Work out the finished part from the listing and answer in its coordinate system (mm). Face numbers are marked on the shaded views. A direction names the side the tool comes from. Coordinates: 2 decimals unless noted, no trailing zeros. Order: outer loops, then holes, each group sorted by start corner. A loop starts at its lowest first (then second) coordinate and runs counter-clockwise, first axis right, second up. Notation, with made-up numbers: M 31,85 L 87,85 A31 ccw 87,114 Z; hole C 0.5,33.25 d4. An arc over 180 degrees is marked long. Write item = value, one per line. Start each with the question number.
Q1. Determine the mould class of the marked faces 3, 4 and 5 for opening direction X: released by +X, released by -X, zero draft, split by the parting line, or undercut.
Q2. Find section B-B on z = -11.5. Give the vertices of the cut face in (x, y), and give its area (3 significant figures).
Q3. Find section A-A on y = 11. Give the vertices of the cut face in (x, z), and give its area (3 significant figures).
Q4. A tool of negligible diameter and unlimited length cuts with its end or side. For the marked faces 1 and 2, from which of +Z, -Z, +X, -X, +Y, -Y can it reach the whole face along a straight path? Write none if from no direction.
Q5. Find section C-C on x = 5.25. Give the vertices of the cut face in (y, z), and give its area (3 significant figures).
Q6. Straight lines are drawn through the part: line 1 along X through (y, z) = (15, -10.75); line 2 along Z through (x, y) = (4.5, 17.25); line 3 along Y through (x, z) = (9.25, -7.5). For each, find the intervals that lie inside material, in ascending order.
Q7. This flat-tipped pin is pushed along its axis until it touches: P1, Ø1.5, axis at x = 4, y = 3, coming from the +Z side. Where does it stop, or does it pass through?
Q8. Find section D-D on x = 2.75. Give the vertices of the cut face in (y, z), and give its area (3 significant figures).
```python
from build123d import *

# Parameters (mm, degrees)
SKETCH1_W           = 12
SKETCH1_H           = 16
BOSS_EXTRUDE1_DEPTH = 18
SHELL1_T            = -2
SKETCH2_R           = 0.75
CUT_EXTRUDE1_DEPTH  = 10


with BuildPart() as part:
    # Sketch1 → Boss-Extrude1 (new body)
    with BuildSketch(Plane(origin=(0, 0, 0), x_dir=(1, 0, 0), z_dir=(0, 1, 0))):
        with Locations((6, 8)):
            Rectangle(SKETCH1_W, SKETCH1_H)
    extrude(amount=BOSS_EXTRUDE1_DEPTH)

    # Shell1
    shell1_openings = [part.faces().sort_by_distance(p)[0] for p in [
        (6, 18, -8),
    ]]
    offset(amount=SHELL1_T, openings=shell1_openings, kind=Kind.INTERSECTION)

    # Sketch2 → Cut-Extrude1 (cut)
    with BuildSketch(Plane.XZ):
        with Locations((4.770114722, -4.163836206)):
            Circle(SKETCH2_R)
        with Locations((4.770114722, -6.703836206)):
            Circle(SKETCH2_R)
        with Locations((4.770114721, -11.783836206)):
            Circle(SKETCH2_R)
    extrude(amount=-CUT_EXTRUDE1_DEPTH, mode=Mode.SUBTRACT)


solid = part.part
```
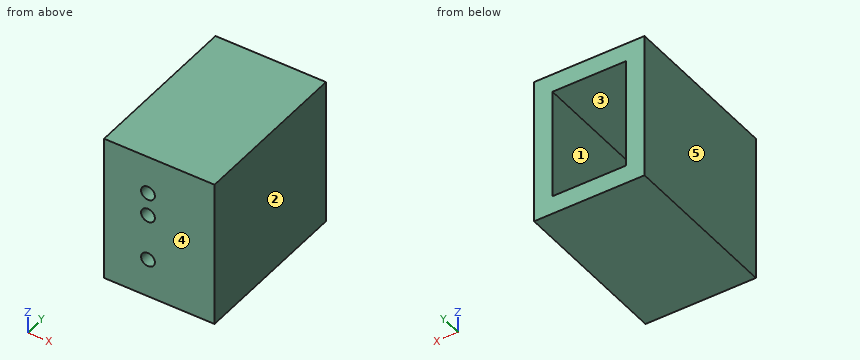
Findings below:
q1.face_3 = undercut
q1.face_4 = zero draft
q1.face_5 = released by -X
q2.outline = M 0,0 L 4.08,0 L 4.08,2 L 2,2 L 2,18 L 0,18 Z; M 5.46,0 L 12,0 L 12,18 L 10,18 L 10,2 L 5.46,2 Z
q2.area = 85.2 mm^2
q3.outline = M 0,-16 L 12,-16 L 12,0 L 0,0 Z; hole M 2,-14 L 10,-14 L 10,-2 L 2,-2 Z
q3.area = 96.0 mm^2
q4.face_1 = +Y
q4.face_2 = +Z, -Z, +X, +Y, -Y
q5.outline = M 0,-16 L 18,-16 L 18,-14 L 2,-14 L 2,-12.36 L 0,-12.36 Z; M 0,-11.21 L 2,-11.21 L 2,-7.28 L 0,-7.28 Z; M 0,-6.13 L 2,-6.13 L 2,-4.74 L 0,-4.74 Z; M 0,-3.59 L 2,-3.59 L 2,-2 L 18,-2 L 18,0 L 0,0 Z
q5.area = 89.1 mm^2
q6.line_1 = 0 to 2, 10 to 12
q6.line_2 = -16 to -14, -2 to 0
q6.line_3 = 0 to 2
q7.P1 = 0
q8.outline = M 0,-16 L 18,-16 L 18,-14 L 2,-14 L 2,-2 L 18,-2 L 18,0 L 0,0 Z
q8.area = 96.0 mm^2
